Work out the finished part from the listing and answer in its coordinate system (mm). A direction names the side the tool comes from. Round coordinates to 2 decimals unless told otherwise and drop trailing zeros. Loops run counter-clockwise (first coordinate to the right, second up) from the corner with the lowest first, then second, coordinate; pieces in that order, holes last. Notation, with made-up numbers: M 20.5,26 L 32.5,26 A32 cw 32.5,63 Z; hole C 29,-36 d2. An arc over 180 degrees is marked long. One line per item, written item: value.
```python
from build123d import *

# Parameters (mm, degrees)
F0_R     = 11
F1_DEPTH = 8.5
F3_DEPTH = 8.5
F5_DEPTH = 8.5


with BuildPart() as f1:
    # F0 (on Right) → F1 (new body)
    with BuildSketch(Plane.YZ):
        Circle(F0_R)
    extrude(amount=F1_DEPTH)

    # F2 (on face) → F3 (cut, through all)
    with BuildSketch(Plane.YZ.offset(8.5)):
        with BuildLine():
            Line((-1, 3), (-1, 7.433034))
            ThreePointArc((-1, 7.433034), (-6.495191, 3.75), (-6.937197, -2.850492))
            Line((-6.937197, -2.850492), (-3.098076, -0.633975))
            Line((-3.098076, -0.633975), (-2.94949, -0.548188))
            ThreePointArc((-2.94949, -0.548188), (-2.598076, 1.5), (-1, 2.828427))
            Line((-1, 2.828427), (-1, 3))
        make_face()
        with BuildLine():
            Line((1, 3.171573), (1, 3))
            Line((1, 3), (1, 2.828427))
            ThreePointArc((1, 2.828427), (2.598076, 1.5), (2.94949, -0.548188))
            Line((2.94949, -0.548188), (3.098076, -0.633975))
            Line((3.098076, -0.633975), (6.937197, -2.850492))
            ThreePointArc((6.937197, -2.850492), (6.495191, 3.75), (1, 7.433034))
            Line((1, 7.433034), (1, 3.171573))
        make_face()
        with BuildLine():
            Line((-1.94949, -2.280239), (-2.098076, -2.366025))
            Line((-2.098076, -2.366025), (-5.937197, -4.582543))
            ThreePointArc((-5.937197, -4.582543), (0, -7.5), (5.937197, -4.582543))
            Line((5.937197, -4.582543), (2.098076, -2.366025))
            Line((2.098076, -2.366025), (1.94949, -2.280239))
            ThreePointArc((1.94949, -2.280239), (0, -3), (-1.94949, -2.280239))
        make_face()
    extrude(amount=-F3_DEPTH, mode=Mode.SUBTRACT)

    # F4 (on face) → F5 (cut, through all)
    with BuildSketch(Plane.YZ.offset(8.5)):
        with BuildLine():
            Line((1.118034, 1), (-1.118034, 1))
            ThreePointArc((-1.118034, 1), (0, -1.5), (1.118034, 1))
        make_face()
    extrude(amount=-F5_DEPTH, mode=Mode.SUBTRACT)


solid = f1.part
```
1) Find section A-A (z = 0). Give the vertices of the cut face in (x, y), then the cut area to 3 significant figures.
Check values:
outline: M 0,-11 L 8.5,-11 L 8.5,-7.5 L 0,-7.5 Z; M 0,-3 L 8.5,-3 L 8.5,-1.5 L 0,-1.5 Z; M 0,1.5 L 8.5,1.5 L 8.5,3 L 0,3 Z; M 0,7.5 L 8.5,7.5 L 8.5,11 L 0,11 Z
area: 85.0 mm2
2) Find section B-B (y = 0). Give the vertices of the cut face in (x, z).
Check values:
outline: M 0,-11 L 8.5,-11 L 8.5,-7.5 L 0,-7.5 Z; M 0,-3 L 8.5,-3 L 8.5,-1.5 L 0,-1.5 Z; M 0,1 L 8.5,1 L 8.5,11 L 0,11 Z
3) For faces 1 (the face through (0, 2, 0)), 2 (the face through (4.3, -2.6, 1.5)), determine the directions among +Z, -Z, +X, -X, +Y, -Y from which every point of the face is accessible in a straight line to the end or side of a thin tool.
Check values:
face 1: +Z, -Z, -X, +Y, -Y
face 2: +X, -X
4) Find the intervals of material crossed by probe 1 along Z at (x, y) = (2.25, -4.5); probe 2 along Y at (x, z) = (0.75, 4); probe 3 along Z at (x, y) = (3.75, 0.25), in increasing order. Write a range as from..to.
Check values:
probe 1: -10.04..-6, -3.75..-1.44, 6..10.04
probe 2: -10.25..-6.34, -1..1, 6.34..10.25
probe 3: -11..-7.5, -2.99..-1.48, 1..11
5) The mould has two halves that part along Z. Classify faces 3 (the face through (4.19, -2.38, -10.74)), 4 (the face through (8.5, 2, 0)), 5 (the face through (4.3, -0.1, -7.5)): +Z half, -Z half, draft (parallel to the pull), parting line (faces both ways), or undercut.
Check values:
face 3: parting line
face 4: draft
face 5: undercut
6) Find section C-C (x = 5). Give the vertices of the cut face in (y, z), then the cut area to 3 significant figures.
Check values:
outline: C 0,0 d22; hole M -6.94,-2.85 L -3.1,-0.63 L -2.95,-0.55 A3 cw -1,2.83 L -1,7.43 A7.5 ccw Z; hole M -5.94,-4.58 A7.5 ccw 5.94,-4.58 L 2.1,-2.37 L 1.95,-2.28 A3 cw -1.95,-2.28 L -2.1,-2.37 Z; hole M -1.12,1 A1.5 ccw long 1.12,1 Z; hole M 1,2.83 A3 cw 2.95,-0.55 L 3.1,-0.63 L 6.94,-2.85 A7.5 ccw 1,7.43 Z
area: 253 mm2
7) Each of these flat-tipped pins is pushed along its axis until it touches: pin 1 (5 mm diameter, centred on x = 4, z = 6, fed in from -Y); pin 2 (4 mm diameter, centred on x = 4.5, z = -1.5, fed in from +Y); pin 3 (5 mm diameter, centred on x = 3.5, z = 4, fed in from +Y); pin 4 (1.5 mm diameter, centred on x = 1.5, y = -4, fed in from +Z). Where does it stop, or does it pass through?
Check values:
pin 1: y = -10.43
pin 2: y = 11
pin 3: y = 10.9
pin 4: z = 10.51
8) Find section D-D (z = -4). Give the vertices of the cut face in (x, y), then the cut area to 3 significant figures.
Check values:
outline: M 0,-10.25 L 8.5,-10.25 L 8.5,-4.93 L 0,-4.93 Z; M 0,4.93 L 8.5,4.93 L 8.5,10.25 L 0,10.25 Z
area: 90.4 mm2
